The model under review builds one solid part; all positions refer to its coordinate system, in mm. A direction names the side the tool comes from. Round coordinates to 2 decimals unless told otherwise and drop trailing zeros. Write each loop counter-clockwise with the first axis right and the second up, starting at its lowest first coordinate (ties: lowest second). Pieces come first, ordered by that corner, then holes. Notation, with made-up numbers: (-34.5, 31.25) - (18.5, 31.25) arc R26 ccw to (18.5, 68.25) - close; hole circle Ø10 at (66.25, 78). An arc over 180 degrees is marked (long way). Return JSON: item names as keys, results as strings.
from build123d import *

# Parameters (mm, degrees)
ESBO_O1_W                = 130
ESBO_O1_H                = 130
RESSALTO_EXTRUS_O1_DEPTH = 44
ESBO_O13_R               = 45
ESBO_O13_R_2             = 40
RESSALTO_EXTRUS_O7_DEPTH = 10
ESBO_O2_R                = 60
ESBO_O2_R_2              = 50
RESSALTO_EXTRUS_O2_DEPTH = 650
ESBO_O3_W                = 130
ESBO_O3_H                = 130
RESSALTO_EXTRUS_O3_DEPTH = 80
ESBO_O4_R                = 8
RESSALTO_EXTRUS_O4_DEPTH = 754
ESBO_O5_R                = 37.5
RESSALTO_EXTRUS_O5_DEPTH = 10
CORTE_EXTRUS_O1_DEPTH    = 10
ESBO_O7_R                = 28.5
CORTE_EXTRUS_O2_DEPTH    = 280
ESBO_O8_W                = 50
ESBO_O8_H                = 100
RESSALTO_EXTRUS_O6_DEPTH = 100
ESBO_O9_R                = 18
CORTE_EXTRUS_O3_DEPTH    = 91
ESBO_O10_R               = 12.25
CORTE_EXTRUS_O4_DEPTH    = 65
ESBO_O11_R               = 12.25
CORTE_EXTRUS_O5_DEPTH    = 65
ESBO_O12_R               = 40
CORTE_EXTRUS_O6_DEPTH    = 22
ESBO_O14_R               = 45
ESBO_O14_R_2             = 40
RESSALTO_EXTRUS_O8_DEPTH = 10


with BuildPart() as part:
    # Esboço1 → Ressalto-extrusão1 (new body)
    with BuildSketch(Plane.XY):
        Rectangle(ESBO_O1_W, ESBO_O1_H)
    extrude(amount=RESSALTO_EXTRUS_O1_DEPTH)

    # Esboço13 → Ressalto-extrusão7 (add)
    with BuildSketch(Plane.XY.offset(44)):
        Circle(ESBO_O13_R)
        Circle(ESBO_O13_R_2, mode=Mode.SUBTRACT)
    extrude(amount=RESSALTO_EXTRUS_O7_DEPTH)

    # Esboço2 → Ressalto-extrusão2 (add)
    with BuildSketch(Plane.XY.offset(44)):
        Circle(ESBO_O2_R)
        Circle(ESBO_O2_R_2, mode=Mode.SUBTRACT)
    extrude(amount=RESSALTO_EXTRUS_O2_DEPTH)

    # Esboço3 → Ressalto-extrusão3 (add)
    with BuildSketch(Plane.XY.offset(694)):
        Rectangle(ESBO_O3_W, ESBO_O3_H)
    extrude(amount=RESSALTO_EXTRUS_O3_DEPTH)

    # Esboço4 → Ressalto-extrusão4 (add)
    with BuildSketch(Plane.XY.offset(44)):
        with Locations((-48.5, 48.5)):
            Circle(ESBO_O4_R)
        with Locations((-48.5, -48.5)):
            Circle(ESBO_O4_R)
        with Locations((48.5, -48.5)):
            Circle(ESBO_O4_R)
        with Locations((48.5, 48.5)):
            Circle(ESBO_O4_R)
    extrude(amount=RESSALTO_EXTRUS_O4_DEPTH)

    # Esboço5 → Ressalto-extrusão5 (add)
    with BuildSketch(Plane.XY.offset(774)):
        Circle(ESBO_O5_R)
    extrude(amount=RESSALTO_EXTRUS_O5_DEPTH)

    # Esboço6 → Corte-extrusão1 (cut)
    with BuildSketch(Plane.XY.offset(784)):
        with BuildLine():
            Line((-35.911089872, 10.800167787), (-27.308764605, 25.699832213))
            ThreePointArc((-27.308764605, 25.699832213), (-32.475952642, 18.75), (-35.911089872, 10.800167787))
        make_face()
        with BuildLine():
            Line((-8.602325267, 36.5), (8.602325267, 36.5))
            ThreePointArc((8.602325267, 36.5), (0, 37.5), (-8.602325267, 36.5))
        make_face()
        with BuildLine():
            Line((27.308764605, 25.699832213), (35.911089872, 10.800167787))
            ThreePointArc((35.911089872, 10.800167787), (32.475952642, 18.75), (27.308764605, 25.699832213))
        make_face()
        with BuildLine():
            ThreePointArc((-35.911089872, -10.800167787), (-32.475952642, -18.75), (-27.308764605, -25.699832213))
            Line((-27.308764605, -25.699832213), (-35.911089872, -10.800167787))
        make_face()
        with BuildLine():
            ThreePointArc((-8.602325267, -36.5), (0, -37.5), (8.602325267, -36.5))
            Line((8.602325267, -36.5), (-8.602325267, -36.5))
        make_face()
        with BuildLine():
            ThreePointArc((27.308764605, -25.699832213), (32.475952642, -18.75), (35.911089872, -10.800167787))
            Line((35.911089872, -10.800167787), (27.308764605, -25.699832213))
        make_face()
    extrude(amount=-CORTE_EXTRUS_O1_DEPTH, mode=Mode.SUBTRACT)

    # Esboço7 → Corte-extrusão2 (cut)
    with BuildSketch(Plane.XY.offset(784)):
        Circle(ESBO_O7_R)
    extrude(amount=-CORTE_EXTRUS_O2_DEPTH, mode=Mode.SUBTRACT)

    # Esboço8 → Ressalto-extrusão6 (add)
    with BuildSketch(Plane(origin=(0, 0, 0), x_dir=(-1, 0, 0), z_dir=(0, 0, -1))):
        Rectangle(ESBO_O8_W, ESBO_O8_H)
    extrude(amount=RESSALTO_EXTRUS_O6_DEPTH)

    # Esboço9 → Corte-extrusão3 (cut, through all)
    with BuildSketch(Plane.ZY.offset(25)):
        with BuildLine():
            Line((-100, 50), (-100, 2.01e-07))
            ThreePointArc((-100, 2.01e-07), (-85.355338988, 35.355339131), (-50, 50))
            Line((-50, 50), (-100, 50))
        make_face()
        with BuildLine():
            Line((-100, -50), (-50, -50))
            ThreePointArc((-50, -50), (-85.355339131, -35.355338988), (-100, 2.01e-07))
            Line((-100, 2.01e-07), (-100, -50))
        make_face()
        with Locations((-50, 0)):
            Circle(ESBO_O9_R)
    extrude(amount=-CORTE_EXTRUS_O3_DEPTH, mode=Mode.SUBTRACT)

    # Esboço10 → Corte-extrusão4 (cut)
    with BuildSketch(Plane(origin=(0, 65, 0), x_dir=(1, 0, 0), z_dir=(0, 1, 0))):
        with Locations((0, -22)):
            Circle(ESBO_O10_R)
    extrude(amount=-CORTE_EXTRUS_O4_DEPTH, mode=Mode.SUBTRACT)

    # Esboço11 → Corte-extrusão5 (cut)
    with BuildSketch(Plane(origin=(0, 65, 0), x_dir=(1, 0, 0), z_dir=(0, 1, 0))):
        with Locations((0, -712)):
            Circle(ESBO_O11_R)
    extrude(amount=-CORTE_EXTRUS_O5_DEPTH, mode=Mode.SUBTRACT)

    # Esboço12 → Corte-extrusão6 (cut)
    with BuildSketch(Plane.XY.offset(44)):
        Circle(ESBO_O12_R)
    extrude(amount=-CORTE_EXTRUS_O6_DEPTH, mode=Mode.SUBTRACT)

    # Esboço14 → Ressalto-extrusão8 (add)
    with BuildSketch(Plane(origin=(0, 0, 694), x_dir=(-1, 0, 0), z_dir=(0, 0, -1))):
        Circle(ESBO_O14_R)
        Circle(ESBO_O14_R_2, mode=Mode.SUBTRACT)
    extrude(amount=RESSALTO_EXTRUS_O8_DEPTH)


solid = part.part
(1) Add section B-B (x = 0). Give the number of separate pieces and of enclosed holes in the cut face, plus the area to 3 significant figures.
Filled in:
{"separate pieces": "3", "enclosed holes": "1", "area": "29,100 mm2"}
(2) Clearance check with flat-ended pins moving along their axes: pin 1 Ø2 at (x, z) = (-1.5, 480) entering from -Y; pin 2 Ø10 at (x, z) = (42, 53.5) entering from +Y; pin 3 Ø6 at (x, z) = (5.5, 594) entering from -Y. State where each tip first meets the part, or that it passes through.
Filled in:
{"pin 1": "stops at y = -60", "pin 2": "stops at y = 56.36", "pin 3": "stops at y = -59.95"}
(3) Add section A-A (z = 625). Write out the cut boundary in (x, y), plus the area to 3 significant figures.
Filled in:
{"outline": "circle Ø120 at (0, 0); circle Ø16 at (-48.5, -48.5); circle Ø16 at (-48.5, 48.5); circle Ø16 at (48.5, -48.5); circle Ø16 at (48.5, 48.5); hole circle Ø100 at (0, 0)", "area": "4,260 mm2"}
(4) Mouldability with a two-part tool opening along Y and no side actions: class faces 1 (the cylindrical face through (42.6, -43.1, 364.4)), 2 (the flat face through (48, -48, 798)), 3 (the flat face through (0, 50, -25)), 4 (the cylindrical face through (-59.94, 2.64, 364.45)) as released by +Y, released by -Y, zero draft, split by the parting line, or undercut.
Filled in:
{"face 1": "undercut", "face 2": "zero draft", "face 3": "released by +Y", "face 4": "undercut"}
(5) For faces 5 (the flat face through (-15, 65, 22)), 6 (the flat face through (-29, -53, 44)), 7 (the cylindrical face through (-54.4, -43.1, 785.8)), 8 (the flat face through (-20, -21, 784)), 9 (the flat face through (25, -1, -27)), list the 3-axis set-ups (+Z, -Z, +X, -X, +Y, -Y) from which the entire face can be reached by the end or side of a thin tool; tool diameter is ignored.
Filled in:
{"face 5": "+Z, -Z, +X, -X, +Y", "face 6": "none", "face 7": "+Z", "face 8": "+Z, +X, -X, +Y, -Y", "face 9": "-Z, +X, +Y, -Y"}
(6) Wall thickness on line 1 (Y direction, x = 0, z = 690.75); line 2 (Z direction, x = 28, y = 18); line 3 (X direction, y = 45, z = 112): over which ranges is each line inside the solid? List them lowest first.
Filled in:
{"line 1": "y = -60 to -50, -45 to -40, 40 to 45, 50 to 60", "line 2": "z = 0 to 22, 694 to 784", "line 3": "x = -55.69 to -41.31, -39.69 to -21.79, 21.79 to 39.69, 41.31 to 55.69"}
